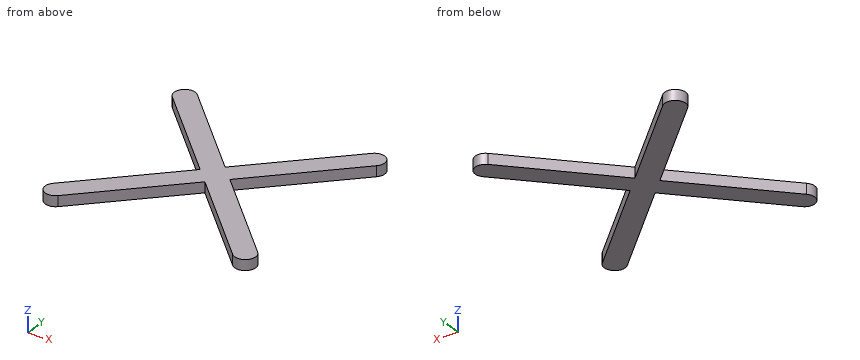
Solid Edge part; units mm, degrees
sketch "Sketch1" plane through (0, 0, 0) normal (0, 0, 1) x (1, 0, 0)
  line L0 (388.9087, 332.3402) -> (-332.3402, -388.9087)
  arc A0 (332.3402, 388.9087) -> (388.9087, 332.3402) centre (360.6245, 360.6245) cw
  line L1 (332.3402, 388.9087) -> (-388.9087, -332.3402)
  arc A1 (-332.3402, -388.9087) -> (-388.9087, -332.3402) centre (-360.6245, -360.6245) cw
  dimension "D1" = 388.9087
extrude "Protrusion1" add sketch "Sketch1" along normal blind 40
mirror "Mirror1" about plane through (0, 0, 0) normal (1, 0, 0) of "Protrusion1"
properties material "Fe 360 B UNI 7070"
Work out the finished part from the listing and answer in its coordinate system (mm). Coordinates: 2 decimals unless noted, no trailing zeros. Write each loop counter-clockwise with the first axis right and the second up, starting at its lowest first coordinate (ties: lowest second). Pieces come first, ordered by that corner, then holes. Notation, with made-up numbers: (57, 5) - (94, 5) arc R13 ccw to (94, 21) - close; hole circle Ø6 at (-8, 14.25). An arc over 180 degrees is marked (long way). Answer as a JSON object with one key per item and string values.
Q1. Find section B-B (y = 171). Write down the section's boundary in (x, z).
Results list:
{"outline": "(-227.57, 0) - (-114.43, 0) - (-114.43, 40) - (-227.57, 40) - close; (114.43, 0) - (227.57, 0) - (227.57, 40) - (114.43, 40) - close"}
Q2. Find section A-A (x = 310). Write down the section's boundary in (y, z).
Results list:
{"outline": "(-366.57, 0) - (-253.43, 0) - (-253.43, 40) - (-366.57, 40) - close; (253.43, 0) - (366.57, 0) - (366.57, 40) - (253.43, 40) - close"}
Q3. Find section D-D (x = -31). Write down the section's boundary in (y, z).
Results list:
{"outline": "(-87.57, 0) - (87.57, 0) - (87.57, 40) - (-87.57, 40) - close"}
Q4. Consider L1, parallel to Y at x = 210, z = 35.5; L2, parallel to Y at x = 227.5, z = 20.5; L3, parallel to X at y = -314, z = 15.5. Determine where each line is inside the solid, lowest interval first. Write a range as from..to.
Results list:
{"L1": "y = -266.57..-153.43, 153.43..266.57", "L2": "y = -284.07..-170.93, 170.93..284.07", "L3": "x = -370.57..-257.43, 257.43..370.57"}
Q5. Given pin 1 Ø1 at (x, z) = (177.5, 10) entering from -Y; pin 2 Ø8 at (y, z) = (70, 4) entering from +X; pin 3 Ø1 at (y, z) = (-131, 17.5) entering from -X, each flat-ended and moving along its own axis, determine where each tip first touches the part or whether it passes through.
Results list:
{"pin 1": "stops at y = -234.57", "pin 2": "stops at x = 130.57", "pin 3": "stops at x = -188.07"}
Q6. Find section C-C (z = 9.5). Write down the section's boundary in (x, y).
Results list:
{"outline": "(-388.91, -332.34) arc R40 ccw to (-332.34, -388.91) - (0, -56.57) - (332.34, -388.91) arc R40 ccw to (388.91, -332.34) - (56.57, 0) - (388.91, 332.34) arc R40 ccw to (332.34, 388.91) - (0, 56.57) - (-332.34, 388.91) arc R40 ccw to (-388.91, 332.34) - (-56.57, 0) - close"}
